Read the model definition and answer for the solid it produces. Units are mm, in the model's axes. A direction names the side the tool comes from. Give positions to 0.01 mm unless a question says otherwise; leave off trailing zeros. Write each loop counter-clockwise with the first axis right and the second up, starting at its lowest first coordinate (ties: lowest second). Pieces come first, ordered by that corner, then holes. Notation, with made-up numbers: (34.25, 70.25) - (84.25, 70.25) arc R20 ccw to (84.25, 105.25) - close; hole circle Ø11 at (65, 24.5). An arc over 180 degrees is marked (long way). Answer as CSV lines item,"result".
```python
from build123d import *

# Parameters (mm, degrees)
SKETCH1_W           = 39
SKETCH1_H           = 50
BOSS_EXTRUDE1_DEPTH = 2
BOSS_EXTRUDE2_DEPTH = 6


with BuildPart() as part:
    # Sketch1 → Boss-Extrude1 (new body)
    with BuildSketch(Plane.XY):
        with Locations((19.5, 25)):
            Rectangle(SKETCH1_W, SKETCH1_H)
    extrude(amount=BOSS_EXTRUDE1_DEPTH)

    # Sketch1<4> → Boss-Extrude2 (add)
    with BuildSketch(Plane.XY):
        Polygon((13.5, 50), (0, 50), (0, 38.094718221), (2, 38.094718221), (2, 48.094718221), (13.5, 48), align=None)
        Polygon((39, 50), (25.5, 50), (25.5, 48.094718221), (37, 48.094718221), (37, 38.094718221), (39, 38.094718221), align=None)
        Polygon((2, 11.905281779), (0, 11.905281779), (0, 0), (9, 0), (9, 2), (2, 2), align=None)
        Polygon((39, 0), (39, 11.905281779), (37, 11.905281779), (37, 2), (30, 2), (30, 0), align=None)
    extrude(amount=BOSS_EXTRUDE2_DEPTH)


solid = part.part
```
(1) A cutting plane is placed at C-C (y = 40.5). Write down the section's boundary in (x, z), and give its area (3 significant figures).
Worked out:
outline,"(0, 0) - (39, 0) - (39, 6) - (37, 6) - (37, 2) - (2, 2) - (2, 6) - (0, 6) - close"
area,"94.0 mm^2"
(2) A cutting plane is placed at D-D (x = 22). Write down the section's boundary in (y, z).
Worked out:
outline,"(0, 0) - (50, 0) - (50, 2) - (0, 2) - close"
(3) A cutting plane is placed at A-A (z = 3.7). Write down the section's boundary in (x, y).
Worked out:
outline,"(0, 0) - (9, 0) - (9, 2) - (2, 2) - (2, 11.91) - (0, 11.91) - close; (0, 38.09) - (2, 38.09) - (2, 48.09) - (13.5, 48) - (13.5, 50) - (0, 50) - close; (25.5, 48.09) - (37, 48.09) - (37, 38.09) - (39, 38.09) - (39, 50) - (25.5, 50) - close; (30, 0) - (39, 0) - (39, 11.91) - (37, 11.91) - (37, 2) - (30, 2) - close"
(4) For faces 1 (the flat face through (25.5, 49, 4)), 2 (the flat face through (30, 1, 4)), 3 (the flat face through (31, 48.095, 4)), 4 (the flat face through (1, 11.905, 4)), determine the directions among +Z, -Z, +X, -X, +Y, -Y from which every point of the face is accessible in a straight line to the end or side of a thin tool.
Worked out:
face 1,"+Z, +Y, -Y"
face 2,"+Z, -Y"
face 3,"+Z"
face 4,"+Z, +X, -X"
(5) The mould has two halves that part along X. Classify faces 5 (the flat face through (13.5, 49, 4)), 6 (the flat face through (0, 24.7, 1.6)), 7 (the flat face through (38, 11.905, 4)): +X half, -X half, draft (parallel to the pull), parting line (faces both ways), or undercut.
Worked out:
face 5,"undercut"
face 6,"-X half"
face 7,"draft"
(6) This flat-tipped pin is pushed along its axis until it touches: P1, Ø11.5, axis at x = 21.5, y = 26.5, coming from the +Z side. Where does it stop, or does it pass through?
Worked out:
P1,"stops at z = 2"
(7) Find the intervals of material crossed by L1, parallel to Y at x = 2.5, z = 3.85; L2, parallel to X at y = 39, z = 5.45; L3, parallel to Z at x = 8, y = 21.5, in increasing order.
Worked out:
L1,"y = 0 to 2, 48.09 to 50"
L2,"x = 0 to 2, 37 to 39"
L3,"z = 0 to 2"
(8) A cutting plane is placed at B-B (x = 32). Write down the section's boundary in (y, z).
Worked out:
outline,"(0, 0) - (50, 0) - (50, 6) - (48.09, 6) - (48.09, 2) - (2, 2) - (2, 6) - (0, 6) - close"
